Could you check a few things on this model? Use its own coordinates, in mm. Face numbers are marked on the shaded views. A direction names the side the tool comes from. Give positions to 0.01 mm unless a question says otherwise; leave off trailing zeros. Loops run counter-clockwise (first coordinate to the right, second up) from the corner with the lowest first, then second, coordinate; pieces in that order, holes last. Notation, with made-up numbers: (66, 84.25) - (117, 84.25) arc R9 ccw to (117, 94.25) - close; hole circle Ø8 at (27, 60). An arc over 180 degrees is marked (long way). Write each question's results on one line, items separated by ' | '. Start each with the question number.
```python
from build123d import *

# Parameters (mm, degrees)
BOSS_EXTRUDE1_DEPTH = 20
CUT_EXTRUDE3_REACH  = 41.302
SKETCH5_R           = 0.25
CUT_EXTRUDE4_REACH  = 42.898
SKETCH3_R           = 1.5
FILLET3_R           = 0.3
SKETCH12_R          = 3.9
BOSS_EXTRUDE3_DEPTH = 6
BOSS_EXTRUDE4_START = 6
SKETCH13_R          = 3.9
BOSS_EXTRUDE4_DEPTH = 6
FILLET4_R           = 0.5
SKETCH14_R          = 3.05
CUT_EXTRUDE5_DEPTH  = 2


with BuildPart() as part:
    # Sketch1 → Boss-Extrude1 (new body)
    with BuildSketch(Plane.XY):
        Polygon((0, 0), (-14, 0), (-14, -11), (4, -11), (4, 30.8), (-14, 30.8), (-14, 19.8), (0, 19.8), align=None)
    extrude(amount=BOSS_EXTRUDE1_DEPTH)

    # Sketch5 → Cut-Extrude3 (cut, up to next)
    with BuildSketch(Plane.XY.offset(20), mode=Mode.PRIVATE) as cut_extrude3_sk1:
        Circle(SKETCH5_R)
    cut_extrude3_tool1 = extrude(cut_extrude3_sk1.sketch, amount=-CUT_EXTRUDE3_REACH, mode=Mode.PRIVATE) & part.part
    # Sketch5 → Cut-Extrude3 (cut, up to next)
    with BuildSketch(Plane.XY.offset(20), mode=Mode.PRIVATE) as cut_extrude3_sk2:
        with Locations((0, 19.8)):
            Circle(SKETCH5_R)
    cut_extrude3_tool2 = extrude(cut_extrude3_sk2.sketch, amount=-CUT_EXTRUDE3_REACH, mode=Mode.PRIVATE) & part.part
    add(cut_extrude3_tool1.solids().sort_by_distance((0, 0, 20))[0], mode=Mode.SUBTRACT)
    add(cut_extrude3_tool2.solids().sort_by_distance((0, 19.8, 20))[0], mode=Mode.SUBTRACT)

    # Sketch3 → Cut-Extrude4 (cut, up to next)
    with BuildSketch(Plane(origin=(4, 0, 0), x_dir=(0, 0, -1), z_dir=(1, 0, 0)), mode=Mode.PRIVATE) as cut_extrude4_sk1:
        with Locations(Location((-5.65, 9.9, 0), (0, 0, 90))):
            Circle(SKETCH3_R)
    cut_extrude4_tool1 = extrude(cut_extrude4_sk1.sketch, amount=-CUT_EXTRUDE4_REACH, mode=Mode.PRIVATE) & part.part
    # Sketch3 → Cut-Extrude4 (cut, up to next)
    with BuildSketch(Plane(origin=(4, 0, 0), x_dir=(0, 0, -1), z_dir=(1, 0, 0)), mode=Mode.PRIVATE) as cut_extrude4_sk2:
        with Locations(Location((-14.35, 9.9, 0), (0, 0, 90))):
            Circle(SKETCH3_R)
    cut_extrude4_tool2 = extrude(cut_extrude4_sk2.sketch, amount=-CUT_EXTRUDE4_REACH, mode=Mode.PRIVATE) & part.part
    add(cut_extrude4_tool1.solids().sort_by_distance((4, 9.9, 5.65))[0], mode=Mode.SUBTRACT)
    add(cut_extrude4_tool2.solids().sort_by_distance((4, 9.9, 14.35))[0], mode=Mode.SUBTRACT)

    # Fillet3
    fillet3_edges = [part.edges().sort_by_distance(p)[0] for p in [
        (0, 0.25, 10),
        (-0.25, 0, 10),
        (0, 19.55, 10),
        (-0.25, 19.8, 10),
    ]]
    fillet(fillet3_edges, radius=FILLET3_R)

    # Sketch12 → Boss-Extrude3 (add)
    with BuildSketch(Plane.XZ.offset(11)):
        with Locations(Location((-5, 10, 0), (0, 0, 270))):
            Circle(SKETCH12_R)
    extrude(amount=BOSS_EXTRUDE3_DEPTH)

    # Sketch13 → Boss-Extrude4 (add)
    with BuildSketch(Plane(origin=(0, 30.8, 0), x_dir=(1, 0, 0), z_dir=(0, 1, 0)).offset(BOSS_EXTRUDE4_START)):
        with Locations(Location((-5, -10, 0), (0, 0, 90))):
            Circle(SKETCH13_R)
    extrude(amount=-BOSS_EXTRUDE4_DEPTH)

    # Fillet4
    fillet4_edges = [part.edges().sort_by_distance(p)[0] for p in [
        (-14, 19.8, 10),
        (-14, 30.8, 10),
        (4, 30.8, 10),
        (4, -11, 10),
        (-14, -11, 10),
        (-14, 0, 10),
    ]]
    fillet(fillet4_edges, radius=FILLET4_R)

    # Sketch14 → Cut-Extrude5 (cut)
    with BuildSketch(Plane(origin=(4, 0, 0), x_dir=(0, 0, -1), z_dir=(1, 0, 0))):
        with Locations(Location((-14.35, 9.9, 0), (0, 0, 90))):
            Circle(SKETCH14_R)
        with Locations(Location((-5.65, 9.9, 0), (0, 0, 90))):
            Circle(SKETCH14_R)
    extrude(amount=-CUT_EXTRUDE5_DEPTH, mode=Mode.SUBTRACT)


solid = part.part
```
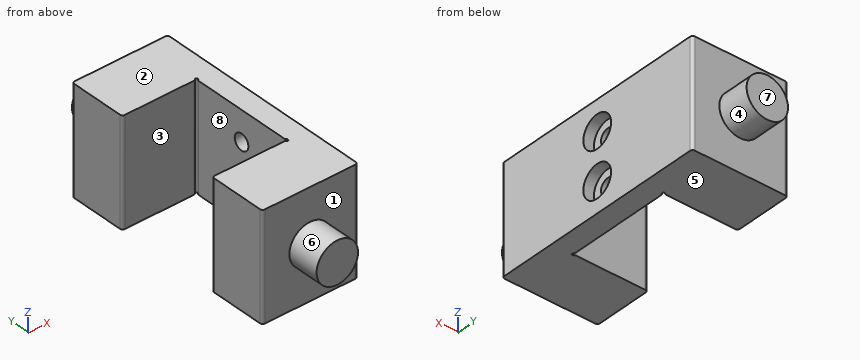
Q1. Which directions (+Z, -Z, +X, -X, +Y, -Y) give clear straight access to the entire face, cutting with the end or side of a thin tool? Please do the marked faces 4, 5, 6, 7 and 8.
Q2. I need wall thicknesses on L1, parallel to Z at x = 3.1, y = 9.9; L2, parallel to Y at x = -7, z = 5.25; L3, parallel to Z at x = 0.6, y = 9.9. Which ranges of each line are inside material? Lowest first, please. Write a range as from..to.
Q3. I want a section at A-A, the plane y = 9.9. List the corners of the cut face in (x, z) for me.
Q4. I want a section at C-C, the plane z = 5. List the corners of the cut face in (x, y) for me.
Q5. If we mould it in two halves opening along Y, with no side actions, what happens to the marked faces 1, 2 and 3? For each: +Y half, -Y half, draft (parallel to the pull), parting line (faces both ways), or undercut.
Q6. I'm going to push flat-ended pins straight in: pin 1 Ø5.5 at (y, z) = (14.5, 8.5) entering from -X; pin 2 Ø2.5 at (y, z) = (9.9, 14.35) entering from +X; pin 3 Ø4 at (x, z) = (-11, 7) entering from +Y; pin 4 Ø5.5 at (y, z) = (9.9, 5.65) entering from +X. Where does each tip first touch, or does it pass through?
Q7. I want a section at B-B, the plane x = -10. List the corners of the cut face in (y, z) for me.
Q8. I want a section at D-D, the plane z = 10. List the corners of the cut face in (x, y) for me, then the cut area to 3 significant figures.
Conclusion:
1) face 4: +Y | face 5: -Z, +X, -X, +Y, -Y | face 6: -Y | face 7: +Z, -Z, +X, -X, +Y | face 8: +Z, -Z, -X
2) L1: 0..2.6, 8.7..11.3, 17.4..20 | L2: -11..0, 19.8..30.8 | L3: 0..4.15, 7.15..12.85, 15.85..20
3) outline: (0, 0) - (4, 0) - (4, 2.6) - (2, 2.6) - (2, 4.15) - (0, 4.15) - close; (0, 7.15) - (2, 7.15) - (2, 8.7) - (4, 8.7) - (4, 11.3) - (2, 11.3) - (2, 12.85) - (0, 12.85) - close; (0, 15.85) - (2, 15.85) - (2, 17.4) - (4, 17.4) - (4, 20) - (0, 20) - close
4) outline: (-14, -10.5) arc R0.5 ccw to (-13.5, -11) - (3.5, -11) arc R0.5 ccw to (4, -10.5) - (4, 6.92) - (2, 6.92) - (2, 8.55) - (0, 8.55) - (0, 0.46) arc R0.3 ccw to (0.14, 0.21) arc R0.25 cw (long way) to (-0.21, -0.14) arc R0.3 ccw to (-0.46, 0) - (-13.5, 0) arc R0.5 ccw to (-14, -0.5) - close; (-14, 20.3) arc R0.5 ccw to (-13.5, 19.8) - (-0.46, 19.8) arc R0.3 ccw to (-0.21, 19.94) arc R0.25 cw (long way) to (0.14, 19.59) arc R0.3 ccw to (0, 19.34) - (0, 11.25) - (2, 11.25) - (2, 12.88) - (4, 12.88) - (4, 30.3) arc R0.5 ccw to (3.5, 30.8) - (-13.5, 30.8) arc R0.5 ccw to (-14, 30.3) - close
5) face 1: -Y half | face 2: draft | face 3: undercut
6) pin 1: x = 0 | pin 2: through | pin 3: y = 30.8 | pin 4: x = 2
7) outline: (-11, 0) - (0, 0) - (0, 20) - (-11, 20) - close; (19.8, 0) - (30.8, 0) - (30.8, 20) - (19.8, 20) - close
8) outline: (-14, -10.5) arc R0.5 ccw to (-13.5, -11) - (-8.9, -11) - (-8.9, -17) - (-1.1, -17) - (-1.1, -11) - (3.5, -11) arc R0.5 ccw to (4, -10.5) - (4, 30.3) arc R0.5 ccw to (3.5, 30.8) - (-1.1, 30.8) - (-1.1, 36.8) - (-8.9, 36.8) - (-8.9, 30.8) - (-13.5, 30.8) arc R0.5 ccw to (-14, 30.3) - (-14, 20.3) arc R0.5 ccw to (-13.5, 19.8) - (-0.46, 19.8) arc R0.3 ccw to (-0.21, 19.94) arc R0.25 cw (long way) to (0.14, 19.59) arc R0.3 ccw to (0, 19.34) - (0, 0.46) arc R0.3 ccw to (0.14, 0.21) arc R0.25 cw (long way) to (-0.21, -0.14) arc R0.3 ccw to (-0.46, 0) - (-13.5, 0) arc R0.5 ccw to (-14, -0.5) - close | area: 568 mm^2
